Can you work these out from the model? Positions are in its coordinate system, mm. A direction names the side the tool comes from. Give positions to 0.01 mm unless a question says otherwise; leave off trailing zeros. Order: outer loops, then holes, each group sorted by start corner. A loop starts at its lowest first (then second) coordinate and runs counter-clockwise, first axis right, second up. Notation, with made-up numbers: (-27, 46) - (-10, 46) arc R19 cw to (-10, 64) - close; hole circle Ø7 at (53.25, 32.25). An arc over 180 degrees is marked (long way). One line per question, with ' | ' between items.
Autodesk Inventor part; units mm, degrees
ref_plane "YZ Plane" through (0, 0, 0) normal (1, 0, 0) x (0, 1, 0)
ref_plane "XZ Plane" through (0, 0, 0) normal (0, 1, 0) x (-1, 0, 0)
ref_plane "XY Plane" through (0, 0, 0) normal (0, 0, 1) x (1, 0, 0)
sketch "Sketch1" plane through (0, 0, 0) normal (0, 1, 0) x (-1, 0, 0)
  line L0 (11.15, 32) -> (-11.15, 32)
  line L1 (-11.15, 32) -> (-11.15, -27)
  line L2 (11.15, -27) -> (11.15, 32)
  line L3 (11.15, 32) -> (-11.15, -32) construction
  line L4 (-11.15, 32) -> (11.15, -32) construction
  arc A0 (6.15, -32) -> (11.15, -27) centre (6.15, -27) ccw
  arc A1 (-11.15, -27) -> (-6.15, -32) centre (-6.15, -27) ccw
  line L5 (2.5547, -34.4) -> (0, -34.4) construction
  circle A2 centre (0, -34.4) radius 1.5
  line L6 (2.6003, -36.8) -> (-2.6003, -36.8)
  line L7 (-2.6003, -36.8) -> (-2.6003, -33)
  line L8 (2.5547, -32) -> (2.6003, -32)
  line L9 (2.6003, -33) -> (2.6003, -36.8)
  line L10 (2.6003, -36.8) -> (-2.6003, -32) construction
  line L11 (-2.6003, -36.8) -> (1.1023, -33.3826) construction
  line L12 (-6.15, -32) -> (-3.6003, -32)
  line L13 (3.6003, -32) -> (6.15, -32)
  arc A3 (3.6003, -32) -> (2.6003, -33) centre (3.6003, -33) ccw
  arc A4 (-2.6003, -33) -> (-3.6003, -32) centre (-3.6003, -33) ccw
  point P0 (0, 0)
  point P1 (0, -32)
  dimension "d19" = 3
  dimension "d14" = 22.3
  dimension "d15" = 64
  dimension "d16" = 5
  dimension "d17" = 5
  dimension "d18" = 2.4
  dimension "d20" = 1
extrude "Extrusion5" add sketch "Sketch1" along normal blind 18.7
sketch "Sketch5" plane through (0, 18.7, 0) normal (0, 1, 0) x (1, 0, 0)
  arc A0 (-6.15, 32) -> (-11.15, 27) centre (-6.15, 27) ccw construction
  line L0 (-11.15, 27) -> (-11.15, -32) construction
  line L1 (-11.15, -32) -> (11.15, -32) construction
  line L2 (11.15, -32) -> (11.15, 27) construction
  arc A1 (11.15, 27) -> (6.15, 32) centre (6.15, 27) ccw construction
  line L3 (6.15, 32) -> (3.6003, 32) construction
  arc A2 (3.6003, 32) -> (2.6003, 33) centre (3.6003, 33) ccw construction
  line L4 (2.6003, 33) -> (2.6003, 36.8) construction
  line L5 (2.6003, 36.8) -> (-2.6003, 36.8) construction
  line L6 (-2.6003, 36.8) -> (-2.6003, 33) construction
  arc A3 (-2.6003, 33) -> (-3.6003, 32) centre (-3.6003, 33) ccw construction
  line L7 (-3.6003, 32) -> (-6.15, 32) construction
  circle A4 centre (0, 34.4) radius 1.5 construction
  line L8 (-3.6003, 32) -> (-6.15, 32) construction
  line L9 (-6.15, 32) -> (-6.15, 20.8) construction
  circle A5 centre (0, 20.8) radius 2.6
  line L10 (0, 0) -> (0, 39.0389) construction
  line L11 (8.75, 32) -> (-8.75, 32) construction
  line L12 (-4.8752, 32) -> (4.8752, 32) construction
  line L13 (8.75, 32) -> (8.75, 0.2) construction
  circle A6 centre (8.75, 0.2) radius 1.5
  line L14 (-8.75, 32) -> (-8.75, 0.2) construction
  circle A7 centre (-8.75, 0.2) radius 1.5
  point P0 (0, 32)
  dimension "d23" = 11.2
  dimension "d24" = 5.2
  dimension "d29" = 17.5
  dimension "d30" = 31.8
  dimension "d31" = 3
  dimension "d32" = 31.8
  dimension "d33" = 3
extrude "Extrusion6" cut sketch "Sketch5" against normal blind 18 contours A6 | A7
extrude "Extrusion7" add sketch "Sketch5" along normal blind 9.3 contours A5
sketch "Sketch6" plane through (0, 18.7, 0) normal (0, 1, 0) x (1, 0, 0)
  circle A0 centre (0, 20.8) radius 2.6 construction
  line L0 (0, 20.8) -> (0, 10.8) construction
  circle A1 centre (0, 10.8) radius 1.5
  point P0 (0, 0)
  dimension "d38" = 10
  dimension "d39" = 3
extrude "Extrusion8" add sketch "Sketch6" along normal blind 2
sketch "Sketch7" plane through (0, 28, -20.8) normal (0, 1, 0) x (1, 0, 0)
  circle A0 centre (0, 0) radius 2.6 construction
  line L0 (1.8, -1.8762) -> (1.8, 1.8762)
  line L1 (-1.8, 1.8762) -> (-1.8, -1.8762)
  line L2 (-1.3648, -2.213) -> (1.3648, 2.213) construction
  line L3 (1.3648, -2.213) -> (-1.3648, 2.213) construction
  arc A1 (-1.8, 1.8762) -> (-1.8, -1.8762) centre (0, 0) ccw
  circle A2 centre (0, 0) radius 2.6
  arc A3 (1.8, -1.8762) -> (1.8, 1.8762) centre (0, 0) ccw
  point P0 (0, -20.8)
extrude "Extrusion9" cut sketch "Sketch7" against normal blind 8 contours L0 A2 | A1 L1
sketch "Sketch8" plane through (0, 28, 0) normal (0, 1, 0) x (1, 0, 0)
  line L0 (-1.8, 22.6762) -> (-1.8, 18.9238) construction
  arc A0 (-1.8, 18.9238) -> (1.8, 18.9238) centre (0, 20.8) ccw construction
  line L1 (1.8, 18.9238) -> (1.8, 22.6762) construction
  arc A1 (1.8, 22.6762) -> (-1.8, 22.6762) centre (0, 20.8) ccw construction
  circle A2 centre (0, 20.8) radius 0.75
  point P0 (0, 0)
  dimension "d45" = 1.5
extrude "Extrusion10" cut sketch "Sketch8" against normal blind 8
sketch "Sketch9" plane through (-11.15, 0, 32) normal (0, 0, 1) x (1, 0, 0)
  line L0 (0, 0) -> (22.3, 0) construction
  line L1 (22.3, 0) -> (22.3, 18.7) construction
  line L2 (0, 18.7) -> (22.3, 18.7) construction
  line L3 (0, 0) -> (0, 18.7) construction
  circle A0 centre (11.15, 9.35) radius 8.75
  line L4 (0, 0) -> (0, 18.7)
  line L5 (0, 0) -> (22.3, 0)
  line L6 (22.3, 0) -> (22.3, 18.7)
  line L7 (22.3, 18.7) -> (0, 18.7)
  line L8 (0, 18.7) -> (0, 0)
  point P0 (11.15, 0)
  dimension "d48" = 17.5
extrude "Extrusion11" cut sketch "Sketch9" against normal blind 20
sketch "Sketch10" plane through (0, 0, 0) normal (0, -1, 0) x (1, 0, 0)
  line L0 (11.15, 12) -> (-11.15, 12)
  line L1 (-11.15, -27) -> (-11.15, 12)
  arc A0 (-11.15, -27) -> (-6.15, -32) centre (-6.15, -27) ccw
  line L2 (-3.6003, -32) -> (-6.15, -32)
  arc A1 (-2.6003, -33) -> (-3.6003, -32) centre (-3.6003, -33) ccw
  line L3 (-2.6003, -36.8) -> (-2.6003, -33)
  line L4 (2.6003, -36.8) -> (-2.6003, -36.8)
  line L5 (2.6003, -33) -> (2.6003, -36.8)
  arc A2 (3.6003, -32) -> (2.6003, -33) centre (3.6003, -33) ccw
  line L6 (6.15, -32) -> (3.6003, -32)
  arc A3 (6.15, -32) -> (11.15, -27) centre (6.15, -27) ccw
  line L7 (11.15, 12) -> (11.15, -27)
  circle A4 centre (0, -34.4) radius 1.5
  arc A5 (-2.6003, -33) -> (-3.6003, -32) centre (-3.6003, -33) ccw
  line L8 (-3.6003, -32) -> (3.6003, -32)
  point P0 (0, 0)
extrude "Extrusion12" cut sketch "Sketch10" against normal blind 8 contours A2 L5 L4 L3 A1 L8
sketch "Sketch11" plane through (0, 18.7, 0) normal (0, 1, 0) x (1, 0, 0)
  circle A0 centre (0, 34.4) radius 1.5
  line L0 (-11.15, -12) -> (11.15, -12)
  line L1 (11.15, -12) -> (11.15, 27)
  arc A1 (11.15, 27) -> (6.15, 32) centre (6.15, 27) ccw
  line L2 (6.15, 32) -> (3.6003, 32)
  arc A2 (2.6003, 33) -> (3.6003, 32) centre (3.6003, 33) ccw
  line L3 (2.6003, 33) -> (2.6003, 36.8)
  line L4 (2.6003, 36.8) -> (-2.6003, 36.8)
  line L5 (-2.6003, 36.8) -> (-2.6003, 33)
  arc A3 (-3.6003, 32) -> (-2.6003, 33) centre (-3.6003, 33) ccw
  line L6 (-3.6003, 32) -> (-6.15, 32)
  arc A4 (-6.15, 32) -> (-11.15, 27) centre (-6.15, 27) ccw
  line L7 (-11.15, 27) -> (-11.15, -12)
  circle A5 centre (-8.75, 0.2) radius 1.5
  circle A6 centre (8.75, 0.2) radius 1.5
  circle A7 centre (0, 20.8) radius 2.6
  circle A8 centre (0, 10.8) radius 1.5
  arc A9 (-3.6003, 32) -> (-2.6003, 33) centre (-3.6003, 33) ccw
  line L8 (-3.6003, 32) -> (3.6003, 32)
  point P0 (0, 0)
extrude "Extrusion13" cut sketch "Sketch11" against normal blind 8 contours A3 L5 L4 L3 A2 L8
properties part number "motor_placeholder"
(1) Imagine slicing it at B-B (z = -34.4). List the corners of the cut face in (x, y) for me.
Answer below:
outline: (-2.6, 8) - (-1.5, 8) - (-1.5, 10.7) - (-2.6, 10.7) - close; (1.5, 8) - (2.6, 8) - (2.6, 10.7) - (1.5, 10.7) - close
(2) If we mould it in two halves opening along X, with no side actions, what happens to faces 6 (the face through (0, 20.7, -11)), 7 (the face through (-10.25, 9.83, -0.27)), 8 (the face through (9.65, 9.22, -30.57))? For each: released by +X, released by -X, zero draft, split by the parting line, or undercut.
Answer below:
face 6: zero draft | face 7: undercut | face 8: released by +X
(3) On a 3-axis mill with a long thin cutter (end or side, diameter ignored), from which of +Z, -Z, +X, -X, +Y, -Y can I reach the whole of each face in a straight line? I mean faces 1 (the face through (-1.8, 24, -21)), 2 (the face through (1.4, 23.28, -18.61)), 3 (the face through (-2, 10.7, -34)), 4 (the face through (-1.9, 0.81, 22.14)), 5 (the face through (-2, 8, -34)). Say none if no direction works.
Answer below:
face 1: +Z, -Z, -X, +Y | face 2: +Y | face 3: -Z, +X, -X, +Y | face 4: +Z | face 5: -Z, +X, -X, -Y
(4) Imagine slicing it at C-C (y = 3.75). List the corners of the cut face in (x, z) for me, and give its area (3 significant figures).
Answer below:
outline: (-11.15, -27) arc R5 ccw to (-6.15, -32) - (6.15, -32) arc R5 ccw to (11.15, -27) - (11.15, 12) - (6.72, 12) - (6.72, 32) - (-6.72, 32) - (-6.72, 12) - (-11.15, 12) - close; hole circle Ø3 at (-8.75, -0.2); hole circle Ø3 at (8.75, -0.2) | area: 1,230 mm^2
(5) If I drill on line 1 (X direction, y = 6.5, z = -0.2); line 2 (Z direction, x = 0, y = 24); line 3 (X direction, y = 9.65, z = -34.4), over which ranges is the centre line in solid material (lowest first)?
Answer below:
line 1: -11.15 to -10.25, -7.25 to 7.25, 10.25 to 11.15 | line 2: -23.4 to -21.55, -20.05 to -18.2 | line 3: -2.6 to -1.5, 1.5 to 2.6
(6) Imagine slicing it at A-A (x = 0). List the corners of the cut face in (y, z) for me.
Answer below:
outline: (0, -32) - (8, -32) - (8, -32.9) - (10.7, -32.9) - (10.7, -32) - (18.7, -32) - (18.7, -23.4) - (28, -23.4) - (28, -21.55) - (20, -21.55) - (20, -20.05) - (28, -20.05) - (28, -18.2) - (18.7, -18.2) - (18.7, -12.3) - (20.7, -12.3) - (20.7, -9.3) - (18.7, -9.3) - (18.7, 12) - (18.1, 12) - (18.1, 32) - (0.6, 32) - (0.6, 12) - (0, 12) - close; (8, -36.8) - (10.7, -36.8) - (10.7, -35.9) - (8, -35.9) - close
(7) Will these pins go through, and if not, where does the flat tip stop? pin 1 (3 mm diameter, centred on y = 9, z = -35.5, fed in from +X); pin 2 (1 mm diameter, centred on x = -0.5, z = -6.5, fed in from +Y); pin 3 (0.9 mm diameter, centred on x = 8.5, z = 0.5, fed in from +Y); pin 4 (2.5 mm diameter, centred on x = 0, z = -34.4, fed in from +Y) (1 decimal).
Answer below:
pin 1: x = 2.6 | pin 2: y = 18.7 | pin 3: y = 0.7 | pin 4: through
(8) Imagine slicing it at D-D (z = -0.2). List the corners of the cut face in (x, y) for me.
Answer below:
outline: (-11.15, 0) - (11.15, 0) - (11.15, 18.7) - (10.25, 18.7) - (10.25, 0.7) - (7.25, 0.7) - (7.25, 18.7) - (-7.25, 18.7) - (-7.25, 0.7) - (-10.25, 0.7) - (-10.25, 18.7) - (-11.15, 18.7) - close
